The model under review builds one solid part; all positions refer to its coordinate system, in mm. A direction names the side the tool comes from. Round coordinates to 2 decimals unless told otherwise and drop trailing zeros. Order: outer loops, then holes, each group sorted by start corner. A loop starts at its lowest first (then second) coordinate and runs counter-clockwise, first axis right, second up. Notation, with made-up numbers: M 60.5,-31 L 101.5,-31 A8 cw 101.5,-23 Z; hole C -39.5,-8.75 d11. An arc over 180 degrees is marked long. Answer as a JSON object with one key per item and string values. Group by question number.
1. Clearance check with flat-ended pins moving along their axes: P1, Ø4, axis at x = -23.5, z = 3.5, coming from the -Y side; P2, Ø5, axis at x = -18, z = 9, coming from the -Y side; P3, Ø6, axis at x = -20, z = 11.5, coming from the -Y side. State where each tip first meets the part, or that it passes through.
2. Add section D-D on x = -24. State the section outline as (y, z) points.
3. Add section A-A on x = -17. State the section outline as (y, z) points.
4. Mouldability with a two-part tool opening along Y and no side actions: class faces 1 (the face through (-33, 13, 6.35)), 2 (the face through (-14.372, 17.437, 6.439)), 3 (the face through (-15.58, 4.63, 6.26)) as released by +Y, released by -Y, zero draft, split by the parting line, or undercut.
5. To check wall thickness, follow probe 1 along X at (y, z) = (14, 11.25) (3 decimals); probe 2 along Y at (x, z) = (-12.5, 10); probe 3 along X at (y, z) = (11.5, 9) (3 decimals). State the ranges of each line that lie inside material, in increasing order. Write a range as [from, to].
6. Machinability: for faces 4 (the face through (-31.456, 7.897, 9.569)), 5 (the face through (-34.664, 13.36, 8.775)), 6 (the face through (-25.4, 23, 3)), which of the approach directions +Z, -Z, +X, -X, +Y, -Y give a long, thin tool a straight path to every point of the face, cutting with its end or side? Answer none if there is none.
7. Add section B-B on z = 8.25. Give the number of separate pieces and of enclosed holes in the cut face, and give its area (3 significant figures).
8. Add section C-C on y = 23.5. State the section outline as (x, z) points.
```python
from build123d import *

# Parameters (mm, degrees)
F1_DEPTH = 12.7
F2_R     = 3.175
F3_DEPTH = 12.7
F3_TAPER = 14
F5_DEPTH = 12.7010001
F6_W     = 38.1
F6_H     = 6.35
F7_DEPTH = 25.401


with BuildPart() as f1:
    # F0 (on Top) → F1 (new body)
    with BuildSketch(Plane.XY):
        with BuildLine():
            ThreePointArc((-25.4, 25.4), (-53.7980633142, 12.7), (-25.4, 0))
            Line((-25.4, 0), (-34.5618496597, 0))
            Line((-34.5618496597, 0), (-34.5618496597, 25.4))
            Line((-34.5618496597, 25.4), (-25.4, 25.4))
        make_face()
        with BuildLine():
            Line((-34.5618496597, 0), (-25.4, 0))
            ThreePointArc((-25.4, 0), (-21.204965459, 5.7439235197), (-19.7203873372, 12.7))
            ThreePointArc((-19.7203873372, 12.7), (-21.204965459, 19.6560764803), (-25.4, 25.4))
            Line((-25.4, 25.4), (-34.5618496597, 25.4))
            Line((-34.5618496597, 25.4), (-34.5618496597, 0))
        make_face()
        with BuildLine():
            ThreePointArc((-19.7203873372, 12.7), (-21.204965459, 5.7439235197), (-25.4, 0))
            ThreePointArc((-25.4, 0), (-15.4225737421, 4.6554132358), (-4.5357142857, 3.0127938932))
            ThreePointArc((-4.5357142857, 3.0127938932), (-1.4778911139, 3.1980667262), (0, 5.8814314849))
            Line((0, 5.8814314849), (0, 19.5185685151))
            ThreePointArc((0, 19.5185685151), (-1.4778911139, 22.2019332738), (-4.5357142857, 22.3872061068))
            ThreePointArc((-4.5357142857, 22.3872061068), (-15.4225737421, 20.7445867642), (-25.4, 25.4))
            ThreePointArc((-25.4, 25.4), (-21.204965459, 19.6560764803), (-19.7203873372, 12.7))
        make_face()
    extrude(amount=F1_DEPTH)

    # F2 (on face) → F3 (cut, through all)
    with BuildSketch(Plane.XY.offset(12.7)):
        with Locations((-36.7592253257, 12.7)):
            Circle(F2_R)
    extrude(amount=-F3_DEPTH, taper=F3_TAPER, mode=Mode.SUBTRACT)

    # F4 (on face) → F5 (cut, through all)
    with BuildSketch(Plane.XY.offset(12.7)):
        with BuildLine():
            ThreePointArc((-25.4, 4.0399547456), (-14.535188109, 7.9500701216), (-3.175, 5.8814314849))
            Line((-3.175, 5.8814314849), (-3.175, 19.5185685151))
            ThreePointArc((-3.175, 19.5185685151), (-14.535188109, 17.4499298784), (-25.4, 21.3600452544))
            Line((-25.4, 21.3600452544), (-30.6912422422, 18.4625566245))
            ThreePointArc((-30.6912422422, 18.4625566245), (-31.4514193427, 17.5192344091), (-31.3248088175, 16.3143710139))
            ThreePointArc((-31.3248088175, 16.3143710139), (-30.4092253257, 12.7), (-31.3248088175, 9.0856289861))
            ThreePointArc((-31.3248088175, 9.0856289861), (-31.4514193427, 7.8807655909), (-30.6912422422, 6.9374433755))
            Line((-30.6912422422, 6.9374433755), (-25.4, 4.0399547456))
        make_face()
        with BuildLine():
            ThreePointArc((-25.4, 25.4), (-53.7980633142, 12.7), (-25.4, 0))
            Line((-25.4, 0), (-43.5066161293, 9.9151979742))
            ThreePointArc((-43.5066161293, 9.9151979742), (-45.1566562358, 12.7), (-43.5066161293, 15.4848020258))
            Line((-43.5066161293, 15.4848020258), (-25.4, 25.4))
        make_face()
    extrude(amount=-F5_DEPTH, mode=Mode.SUBTRACT)

    # F6 (on Front) → F7 (cut, through all)
    with BuildSketch(Plane.XZ):
        with Locations((-44.45, 3.175)):
            Rectangle(F6_W, F6_H)
    extrude(amount=-F7_DEPTH, mode=Mode.SUBTRACT)


solid = f1.part
```
Recorded:
{
 "1": {"P1": "stops at y = 0", "P2": "stops at y = 3.18", "P3": "stops at y = 1.83"},
 "2": {"outline": "M 1.14,0 L 4.94,0 L 4.94,12.7 L 1.14,12.7 Z; M 20.46,0 L 24.26,0 L 24.26,12.7 L 20.46,12.7 Z"},
 "3": {"outline": "M 4.36,0 L 7.61,0 L 7.61,12.7 L 4.36,12.7 Z; M 17.79,0 L 21.04,0 L 21.04,12.7 L 17.79,12.7 Z"},
 "4": {"face 1": "zero draft", "face 2": "undercut", "face 3": "released by -Y"},
 "5": {"probe 1": "x = [-44.878, -39.254], [-34.264, -30.521], [-3.175, 0]", "probe 2": "y = [4.85, 8.03], [17.37, 20.55]", "probe 3": "x = [-44.921, -38.665], [-34.853, -30.505], [-3.175, 0]"},
 "6": {"face 4": "+Z, -Z", "face 5": "+Z", "face 6": "-Z, -X, +Y, -Y"},
 "7": {"separate pieces": "1", "enclosed holes": "2", "area": "403 mm²"},
 "8": {"outline": "M -28.87,6.35 L -25.4,6.35 L -25.4,0 L -22.88,0 L -22.88,12.7 L -28.87,12.7 Z"}
}
